from build123d import *

# Parameters (mm, degrees)
SKETCH_1102_W          = 15.2
SKETCH_1102_H          = 15.2
CUT_EXTRUDE_1177_DEPTH = 34
SKETCH_1232_R          = 2.25
CUT_EXTRUDE_1504_DEPTH = 58.409080292
SKETCH_3_R             = 3.8
SKETCH_3_R_2           = 2.25
CUT_EXTRUDE_1538_DEPTH = 5
CUT_EXTRUDE_2118_DEPTH = 6


with BuildPart() as part:
    # Sketch 450 → Revolve 1 (revolve)
    with BuildSketch(Plane.XY, mode=Mode.PRIVATE) as revolve_1_sk:
        Polygon((3, 43.7), (12.65, 43.7), (12.65, 36.7), (14.15, 36.7), (14.15, 35.2), (16.65, 35.2), (16.65, 8.5), (14.15, 8.5), (14.15, 7), (12.65, 7), (12.65, 0), (0, 0), (0, 30.2), (3, 30.2), align=None)
    revolve(revolve_1_sk.sketch.rotate(Axis((0, 0, 0), (0, 1, 0)), 90), axis=Axis((0, 0, 0), (0, 1, 0)))

    # Sketch 1102 → Cut-Extrude 1177 (cut)
    with BuildSketch(Plane(origin=(0, 0, 0), x_dir=(-1, 0, 0), z_dir=(0, -1, 0))):
        Rectangle(SKETCH_1102_W, SKETCH_1102_H)
    extrude(amount=-CUT_EXTRUDE_1177_DEPTH, mode=Mode.SUBTRACT)

    # Sketch 1232 → Cut-Extrude 1504 (cut, through all)
    with BuildSketch(Plane(origin=(16.65, 0, 0), x_dir=(0, 0, -1), z_dir=(1, 0, 0))):
        with Locations((0, 29.7)):
            Circle(SKETCH_1232_R)
        with Locations((0, 14.7)):
            Circle(SKETCH_1232_R)
    extrude(amount=-CUT_EXTRUDE_1504_DEPTH, mode=Mode.SUBTRACT)

    # Sketch 3 → Cut-Extrude 1538 (cut)
    # profile 1 of 2: a face of its own
    with BuildSketch(Plane(origin=(16.65, 0, 0), x_dir=(0, 0, -1), z_dir=(1, 0, 0))):
        with Locations((0, 29.7)):
            Circle(SKETCH_3_R)
        with Locations((0, 29.7)):
            Circle(SKETCH_3_R_2, mode=Mode.SUBTRACT)
    # profile 2 of 2: a face of its own
    with BuildSketch(Plane(origin=(16.65, 0, 0), x_dir=(0, 0, -1), z_dir=(1, 0, 0))):
        with Locations((0, 14.7)):
            Circle(SKETCH_3_R)
        with Locations((0, 14.7)):
            Circle(SKETCH_3_R_2, mode=Mode.SUBTRACT)
    extrude(amount=-CUT_EXTRUDE_1538_DEPTH, mode=Mode.SUBTRACT)

    # Sketch 1662 → Cut-Extrude 2118 (cut)
    with BuildSketch(Plane.ZY.offset(16.65)):
        Polygon((0, 33.799186911), (3.55, 31.749593456), (3.55, 27.650406544), (0, 25.600813089), (-3.55, 27.650406544), (-3.55, 31.749593456), align=None)
        Polygon((0, 18.799186911), (3.55, 16.749593456), (3.55, 12.650406544), (0, 10.600813089), (-3.55, 12.650406544), (-3.55, 16.749593456), align=None)
    extrude(amount=-CUT_EXTRUDE_2118_DEPTH, mode=Mode.SUBTRACT)


solid = part.part
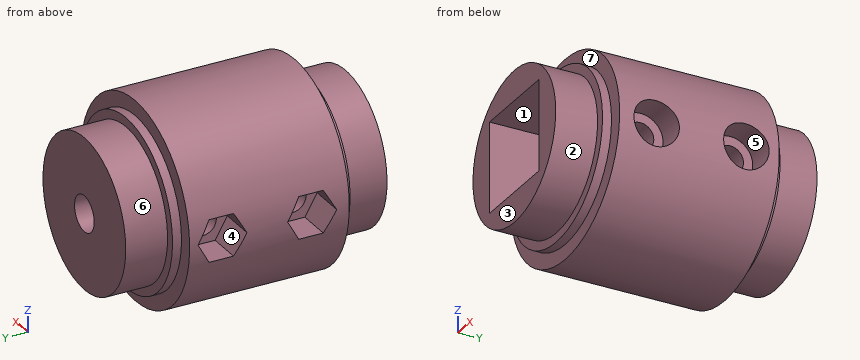
Could you check a few things on this model? Use its own coordinates, in mm. Face numbers are marked on the shaded views. A direction names the side the tool comes from. Give positions to 0.01 mm unless a question says otherwise; leave off trailing zeros. Order: outer loops, then holes, each group sorted by start corner. A loop starts at its lowest first (then second) coordinate and runs counter-clockwise, first axis right, second up.
1. Will these pins go through, and if not, where does the flat tip stop? P1, Ø7.5, axis at x = 1.5, y = 9.5, coming from the +Z side; P2, Ø5, axis at y = 14.7, z = 0, coming from the -X side; P3, Ø4, axis at x = -7.5, y = 28.5, coming from the -Z side; P4, Ø4, axis at x = 10, y = 27.5, coming from the -Z side.
2. Suppose I cut it at A-A (x = 0). List the corners of the cut face in (y, z) for me, plus the area to 3 significant figures.
3. For the marked faces 4, 5, 6 and 7, which set-ups out of +Z, -Z, +X, -X, +Y, -Y let a thin tool reach every point of the face, with its end or its side?
4. We'd pull the mould along X, two halves only. Please class the marked faces 1, 2 and 3: pulls with the +X half, pulls with the -X half, needs draft (parallel to the pull), parting line crosses it, or undercut.
5. I need wall thicknesses on L1, parallel to Y at x = 15, z = 0; L2, parallel to Y at x = -8.8, z = 0; L3, parallel to X at y = 37.5, z = 0. Which ranges of each line are inside material? Lowest first, please.
6. Suppose I cut it at B-B (y = 24). List the corners of the cut face in (x, z) for me, plus the area to 3 significant figures.
7. Suppose I cut it at D-D (y = 29.7). List the corners of the cut face in (x, z) for me.
8. Suppose I cut it at C-C (z = 9.5). List the corners of the cut face in (x, y) for me, plus the area to 3 significant figures.
Solved:
1. P1: stops at z = 16.65
1. P2: stops at x = -10.65
1. P3: stops at z = -15.72
1. P4: stops at z = -14.6
2. outline: (0, -12.65) - (7, -12.65) - (7, -14.15) - (8.5, -14.15) - (8.5, -16.65) - (35.2, -16.65) - (35.2, -14.15) - (36.7, -14.15) - (36.7, -12.65) - (43.7, -12.65) - (43.7, -3) - (34, -3) - (34, -7.6) - (0, -7.6) - close; (0, 7.6) - (34, 7.6) - (34, 3) - (43.7, 3) - (43.7, 12.65) - (36.7, 12.65) - (36.7, 14.15) - (35.2, 14.15) - (35.2, 16.65) - (8.5, 16.65) - (8.5, 14.15) - (7, 14.15) - (7, 12.65) - (0, 12.65) - close
2. area: 753 mm2
3. face 4: -X
3. face 5: +X
3. face 6: +Y
3. face 7: -Y
4. face 1: undercut
4. face 2: parting line crosses it
4. face 3: needs draft
5. L1: y = 8.5 to 10.9, 18.5 to 25.9, 33.5 to 35.2
5. L2: y = 0 to 12.45, 16.95 to 27.45, 31.95 to 43.7
5. L3: x = -12.65 to -3, 3 to 12.65
6. outline: circle Ø33.3 at (0, 0); hole (-7.6, -7.6) - (7.6, -7.6) - (7.6, 7.6) - (-7.6, 7.6) - close
6. area: 640 mm2
7. outline: (-16.27, -3.55) arc R16.65 ccw to (16.21, -3.8) - (11.65, -3.8) - (11.65, -2.25) - (7.6, -2.25) - (7.6, -7.6) - (-7.6, -7.6) - (-7.6, -2.25) - (-10.65, -2.25) - (-10.65, -3.55) - close; (-16.27, 3.55) - (-10.65, 3.55) - (-10.65, 2.25) - (-7.6, 2.25) - (-7.6, 7.6) - (7.6, 7.6) - (7.6, 2.25) - (11.65, 2.25) - (11.65, 3.8) - (16.21, 3.8) arc R16.65 ccw to start
8. outline: (-13.67, 8.5) - (-10.49, 8.5) - (-10.49, 7) - (-8.35, 7) - (-8.35, 0) - (8.35, 0) - (8.35, 7) - (10.49, 7) - (10.49, 8.5) - (13.67, 8.5) - (13.67, 35.2) - (10.49, 35.2) - (10.49, 36.7) - (8.35, 36.7) - (8.35, 43.7) - (-8.35, 43.7) - (-8.35, 36.7) - (-10.49, 36.7) - (-10.49, 35.2) - (-13.67, 35.2) - close
8. area: 1,030 mm2
